```python
from build123d import *

# Parameters (mm, degrees)
F2_R     = 2.38125
F3_DEPTH = 25.4
F4_R     = 2.38125
F5_DEPTH = 25.4


with BuildPart() as f1:
    # F0 (on Front) → F1 (revolve)
    with BuildSketch(Plane.XZ):
        with BuildLine():
            Line((0, 12.985748), (0, -40.036752))
            Line((0, -40.036752), (11.364976, -40.036752))
            ThreePointArc((11.364976, -40.036752), (11.813989, -39.850765), (11.999976, -39.401752))
            Line((11.999976, -39.401752), (11.999976, 23.463248))
            Line((11.999976, 23.463248), (11.24966, 23.463248))
            Line((11.24966, 23.463248), (11.24966, 28.543248))
            Line((11.24966, 28.543248), (11.999976, 28.543248))
            Line((11.999976, 28.543248), (11.999976, 37.623748))
            Line((11.999976, 37.623748), (11.237976, 38.385748))
            Line((11.237976, 38.385748), (5.5372, 38.385748))
            ThreePointArc((5.5372, 38.385748), (4.998385, 38.162564), (4.7752, 37.623748))
            Line((4.7752, 37.623748), (4.7752, 12.985748))
            Line((4.7752, 12.985748), (0, 12.985748))
        make_face()
    revolve(axis=Axis((0, 0, -13.525502), (0, 0, -1)))

    # F2 (on Front) → F3 (cut)
    with BuildSketch(Plane.XZ):
        with Locations((0, 26.139926)):
            Circle(F2_R)
    extrude(amount=F3_DEPTH, mode=Mode.SUBTRACT)

    # F4 (on Right) → F5 (cut)
    with BuildSketch(Plane.YZ):
        with Locations((0, 26.043008)):
            Circle(F4_R)
    extrude(amount=F5_DEPTH, mode=Mode.SUBTRACT)


solid = f1.part
```
The model under review builds one solid part; all positions refer to its coordinate system, in mm. A direction names the side the tool comes from. Round coordinates to 2 decimals unless told otherwise and drop trailing zeros. Write each loop counter-clockwise with the first axis right and the second up, starting at its lowest first coordinate (ties: lowest second). Pieces come first, ordered by that corner, then holes. Notation, with made-up numbers: (-36.75, -5.75) - (17.25, -5.75) arc R11 cw to (17.25, 13.25) - close; hole circle Ø6 at (-32.75, -25.75). An arc over 180 degrees is marked (long way). Use one line per item in the form item = value.
Q1. Tool access review of faces 1 (the cylindrical face through (-1.56, -11.9, 33.15)), 2 (the flat face through (3, -11, 23.463)), 3 (the cylindrical face through (-3.789, 2.906, 25.132)): name each direction out of +Z, -Z, +X, -X, +Y, -Y from which nothing blocks a thin tool from reaching the whole face with its end or side.
Answer key:
face_1 = +Z, -Z
face_2 = none
face_3 = +Z
Q2. Consider section B-B (y = 0). State the section outline as (x, z) points (3 decimals), and give its area (3 significant figures).
Answer key:
outline = (-12, -39.402) arc R0.635 ccw to (-11.365, -40.037) - (11.365, -40.037) arc R0.635 ccw to (12, -39.402) - (12, 23.463) - (11.25, 23.463) - (11.25, 23.662) - (4.775, 23.662) - (4.775, 12.986) - (-4.775, 12.986) - (-4.775, 37.624) arc R0.762 ccw to (-5.537, 38.386) - (-11.238, 38.386) - (-12, 37.624) - (-12, 28.543) - (-11.25, 28.543) - (-11.25, 23.463) - (-12, 23.463) - close; (4.775, 28.424) - (11.25, 28.424) - (11.25, 28.543) - (12, 28.543) - (12, 37.624) - (11.238, 38.386) - (5.537, 38.386) arc R0.762 ccw to (4.775, 37.624) - close
area = 1,600 mm2
Q3. For line 1 (Z direction, x = 0, y = -5.75); line 2 (Z direction, x = 6, y = 0); line 3 (Z direction, x = 2.5, y = 2.5), list the stretches that pass through material, from the lowest coordinate up. Write a range as [from, to].
Answer key:
line_1 = [-40.04, 23.76], [28.52, 38.39]
line_2 = [-40.04, 23.66], [28.42, 38.39]
line_3 = [-40.04, 12.99]
Q4. Consider section A-A (x = 0). State the section outline as (y, z) points (3 decimals).
Answer key:
outline = (-12, -39.402) arc R0.635 ccw to (-11.365, -40.037) - (11.365, -40.037) arc R0.635 ccw to (12, -39.402) - (12, 23.463) - (11.25, 23.463) - (11.25, 28.543) - (12, 28.543) - (12, 37.624) - (11.238, 38.386) - (5.537, 38.386) arc R0.762 ccw to (4.775, 37.624) - (4.775, 12.986) - (-4.775, 12.986) - (-4.775, 23.759) - (-11.25, 23.759) - (-11.25, 23.463) - (-12, 23.463) - close; (-12, 28.543) - (-11.25, 28.543) - (-11.25, 28.521) - (-4.775, 28.521) - (-4.775, 37.624) arc R0.762 ccw to (-5.537, 38.386) - (-11.238, 38.386) - (-12, 37.624) - close
Q5. Consider section C-C (z = 1). State the section outline as (x, y) points.
Answer key:
outline = circle Ø24 at (0, 0)
Q6. Draft analysis for pull direction X (two halves, no side actions). For faces 4 (the cylindrical face through (-1.56, -11.9, -7.53)), 5 (the cylindrical face through (-2.38, -7.65, 26.24)), 6 (the cylindrical face through (7.64, -2.38, 26.15)), state which applies: +X half, -X half, draft (parallel to the pull), parting line (faces both ways), or undercut.
Answer key:
face_4 = parting line
face_5 = undercut
face_6 = draft
Q7. Insertion check: pin 1 Ø10 at (y, z) = (-7.5, 15.5) entering from +X; pin 2 Ø1.5 at (y, z) = (9, -24) entering from +X; pin 3 Ø4 at (x, z) = (8.5, 4) entering from +Y. Each pin has a flat end and moves straight along its axis. Give the tip position at first contact, or say it passes through.
Answer key:
pin_1 = 11.74
pin_2 = 8.71
pin_3 = 10.09
